```python
from build123d import *

# Parameters (mm, degrees)
F0_R     = 17.5
F1_DEPTH = 27.5
F2_R     = 8.5
F3_DEPTH = 120
F4_R     = 5
F5_R     = 3


with BuildPart() as f1:
    # F0 (on Front) → F1 (new body, symmetric)
    with BuildSketch(Plane.XZ):
        Circle(F0_R)
    extrude(amount=F1_DEPTH, both=True)

    # F2 (on Top) → F3 (join)
    with BuildSketch(Plane.XY):
        Circle(F2_R)
    extrude(amount=-F3_DEPTH)

    # F4
    f4_edges = [f1.edges().sort_by_distance(p)[0] for p in [
        (-17.5, 27.5, 0),
        (-17.5, -27.5, 0),
    ]]
    fillet(f4_edges, radius=F4_R)

    # F5
    f5_edges = [f1.edges().sort_by_distance(p)[0] for p in [
        (-8.5, 0, -120),
    ]]
    fillet(f5_edges, radius=F5_R)


solid = f1.part
```
CAD build for the part. Positions are in the model's coordinates, mm. A direction names the side the tool comes from. Give positions to 0.01 mm unless a question says otherwise; leave off trailing zeros. Write each loop counter-clockwise with the first axis right and the second up, starting at its lowest first coordinate (ties: lowest second). Pieces come first, ordered by that corner, then holes. Notation, with made-up numbers: (-27.75, 56.25) -> (-21.75, 56.25) arc R15 cw to (-21.75, 85.25) -> close; hole circle Ø10 at (64, 66). An arc over 180 degrees is marked (long way). Write each question's results on one line, items separated by ' | '.
1. Cut at B-B, the plane y = 0. Write the cut outline in (x, z), then the cut area to 3 significant figures.
Geometry check:
outline: (-8.5, -117) arc R3 ccw to (-5.5, -120) -> (5.5, -120) arc R3 ccw to (8.5, -117) -> (8.5, -15.3) arc R17.5 ccw (long way) to (-8.5, -15.3) -> close | area: 2,710 mm²
2. Which spindle directions (+Z, -Z, +X, -X, +Y, -Y) get a long thin tool onto all of the face, cutting with end or side? Do faces 1 (the flat face through (0, -27.5, 0)), 2 (the cylindrical face through (4.57, 7.167, -65.437)). Say none if no direction does.
Geometry check:
face 1: +Z, -Z, +X, -X, -Y | face 2: -Z
3. Wall check: probe 1 along Y at (x, z) = (7, 10.5); probe 2 along Z at (x, y) = (-3, -17.5); probe 3 along X at (y, z) = (6, -4). Give the ranges that are in metal, low to high. Write a range as [from, to].
Geometry check:
probe 1: [-27.5, 27.5] | probe 2: [-17.24, 17.24] | probe 3: [-17.04, 17.04]
4. Cut at A-A, the plane x = 0. Write the cut outline in (y, z), then the cut area to 3 significant figures.
Geometry check:
outline: (-27.5, -12.5) arc R5 ccw to (-22.5, -17.5) -> (-8.5, -17.5) -> (-8.5, -117) arc R3 ccw to (-5.5, -120) -> (5.5, -120) arc R3 ccw to (8.5, -117) -> (8.5, -17.5) -> (22.5, -17.5) arc R5 ccw to (27.5, -12.5) -> (27.5, 12.5) arc R5 ccw to (22.5, 17.5) -> (-22.5, 17.5) arc R5 ccw to (-27.5, 12.5) -> close | area: 3,640 mm²
5. Cut at C-C, the plane z = -85.5. Write the cut outline in (x, y).
Geometry check:
outline: circle Ø17 at (0, 0)
6. Cut at D-D, the plane y = -14. Write the cut outline in (x, z).
Geometry check:
outline: circle Ø35 at (0, 0)
7. Drop flat-ended pins along their axis: P1, Ø2, axis at x = 0, y = 8, coming from the -Z side; P2, Ø8, axis at y = -15, z = -20, coming from the +X side; P3, Ø4, axis at y = 5.5, z = -63.5, coming from the +X side. Give the stop position or say it passes through.
Geometry check:
P1: z = -119.6 | P2: x = 7.09 | P3: x = 7.75
